Design review of the part shown in the three views and the two pictorial views. Dimensions are in mm from the part's minimum x, y and z. A direction names the side the tool comes from. Give positions to 0.01 mm unless a question says otherwise; leave off trailing zeros. Loops run counter-clockwise (first coordinate to the right, second up) from the corner with the lowest first, then second, coordinate; pieces in that order, holes last.
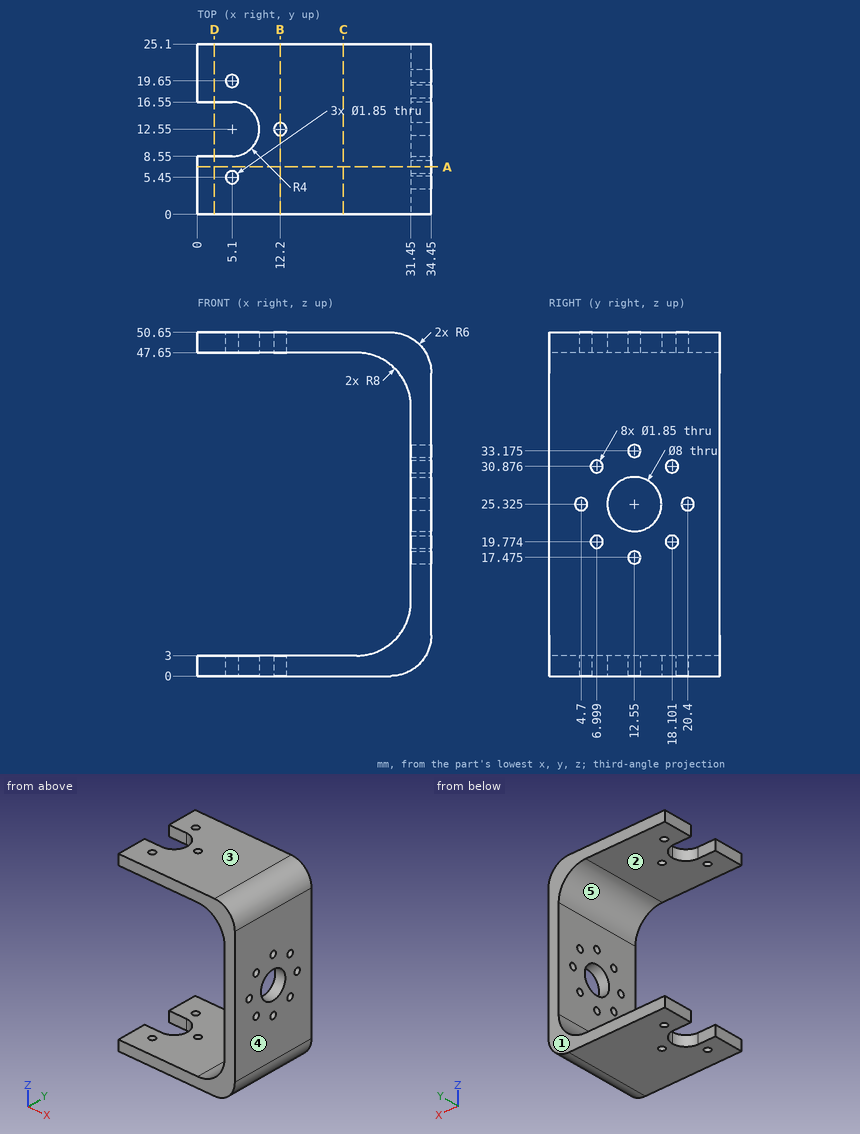
Q1. Machinability: for the marked faces 1 and 2, which of the approach directions +Z, -Z, +X, -X, +Y, -Y give a long, thin tool a straight path to every point of the face, cutting with its end or side? Answer none if there is none.
Answers:
face 1: +Z, -Z, +X, -X, +Y
face 2: -X, +Y, -Y
Q2. For pin 1 Ø1.1 at (x, y) = (5.1, 5.45) entering from +Z; pin 2 Ø1 at (y, z) = (6.5, 35.5) entering from -X, all flat-tipped, find the tip position at first contact; note any pin that passes through.
Answers:
pin 1: passes through
pin 2: stops at x = 31.45
Q3. Consider section B-B on x = 12.2. Give the boundary of the cut face in (y, z) (3 decimals).
Answers:
outline: (0, 0) - (11.625, 0) - (11.625, 3) - (0, 3) - close; (0, 47.65) - (11.625, 47.65) - (11.625, 50.65) - (0, 50.65) - close; (13.475, 0) - (25.1, 0) - (25.1, 3) - (13.475, 3) - close; (13.475, 47.65) - (25.1, 47.65) - (25.1, 50.65) - (13.475, 50.65) - close
Q4. Consider section C-C on x = 21.5. Give the boundary of the cut face in (y, z), plus the area to 3 significant figures.
Answers:
outline: (0, 0) - (25.1, 0) - (25.1, 3) - (0, 3) - close; (0, 47.65) - (25.1, 47.65) - (25.1, 50.65) - (0, 50.65) - close
area: 151 mm2
Q5. Consider section D-D on x = 2.5. Give the boundary of the cut face in (y, z).
Answers:
outline: (0, 0) - (8.55, 0) - (8.55, 3) - (0, 3) - close; (0, 47.65) - (8.55, 47.65) - (8.55, 50.65) - (0, 50.65) - close; (16.55, 0) - (25.1, 0) - (25.1, 3) - (16.55, 3) - close; (16.55, 47.65) - (25.1, 47.65) - (25.1, 50.65) - (16.55, 50.65) - close
Q6. For probe 1 along Z at (x, y) = (15, 14.5); probe 2 along X at (y, z) = (11, 37); probe 3 along Z at (x, y) = (30, 17) (1 decimal), list the stretches that pass through material, from the lowest coordinate up.
Answers:
probe 1: z = 0 to 3, 47.65 to 50.65
probe 2: x = 31.45 to 34.45
probe 3: z = 0.2 to 6.4, 44.2 to 50.4
Q7. Consider section A-A on y = 7. Give the boundary of the cut face in (x, z).
Answers:
outline: (0, 0) - (28.45, 0) arc R6 ccw to (34.45, 6) - (34.45, 18.85) - (31.45, 18.85) - (31.45, 11) arc R8 cw to (23.45, 3) - (0, 3) - close; (0, 47.65) - (23.45, 47.65) arc R8 cw to (31.45, 39.65) - (31.45, 31.8) - (34.45, 31.8) - (34.45, 44.65) arc R6 ccw to (28.45, 50.65) - (0, 50.65) - close; (31.45, 20.7) - (34.45, 20.7) - (34.45, 29.95) - (31.45, 29.95) - close
Q8. Mouldability with a two-part tool opening along Z and no side actions: class the marked faces 3, 4 and 5 as +Z half, -Z half, draft (parallel to the pull), parting line (faces both ways), or undercut.
Answers:
face 3: +Z half
face 4: draft
face 5: undercut
